```python
from build123d import *

# Parameters (mm, degrees)
SKETCH1_W           = 50
SKETCH1_H           = 40
BOSS_EXTRUDE1_DEPTH = 10
SKETCH5_W           = 6
SKETCH5_H           = 5
BOSS_EXTRUDE3_DEPTH = 10
SKETCH6_R           = 2
CUT_EXTRUDE1_DEPTH  = 20
SKETCH8_W           = 10
SKETCH8_H           = 40
CUT_EXTRUDE2_DEPTH  = 25
SKETCH9_W           = 10
SKETCH9_H           = 6
SKETCH9_R           = 1.25
BOSS_EXTRUDE4_DEPTH = 5
SKETCH10_W          = 10
SKETCH10_H          = 5
CUT_EXTRUDE3_DEPTH  = 15
SKETCH11_W          = 5
SKETCH11_H          = 5
BOSS_EXTRUDE5_DEPTH = 10
SKETCH12_R          = 1.25
CUT_EXTRUDE4_DEPTH  = 10
CUT_EXTRUDE5_DEPTH  = 10
CUT_EXTRUDE6_DEPTH  = 10
SCALE1_SCALE        = 2
SKETCH15_W          = 33.464905159
SKETCH15_H          = 55
SKETCH15_W_2        = 35
SKETCH15_H_2        = 25
CUT_EXTRUDE7_DEPTH  = 30


with BuildPart() as part:
    # Sketch1 → Boss-Extrude1 (new body)
    with BuildSketch(Plane(origin=(669.84184187, 0, 0), x_dir=(1, 0, 0), z_dir=(0, 0, 1))):
        with Locations((-671.310344828, 437.637931034)):
            Rectangle(SKETCH1_W, SKETCH1_H)
    boss_extrude1 = extrude(amount=BOSS_EXTRUDE1_DEPTH)

    # Sketch5 → Boss-Extrude3 (add)
    with BuildSketch(Plane(origin=(23.531497042, 0, 0), x_dir=(0, 0, -1), z_dir=(1, 0, 0))):
        with Locations((-5, 442.637931034)):
            Rectangle(SKETCH5_W, SKETCH5_H)
        with Locations((-5, 432.637931034)):
            Rectangle(SKETCH5_W, SKETCH5_H)
    extrude(amount=BOSS_EXTRUDE3_DEPTH)

    # Sketch6 → Cut-Extrude1 (cut)
    with BuildSketch(Plane(origin=(669.84184187, 445.137931034, 0), x_dir=(1, 0, 0), z_dir=(0, 1, 0))):
        with Locations(Location((-641.310344828, -5, 0), (0, 0, 180))):
            Circle(SKETCH6_R)
    extrude(amount=-CUT_EXTRUDE1_DEPTH, mode=Mode.SUBTRACT)

    # Sketch8 → Cut-Extrude2 (cut)
    with BuildSketch(Plane.ZY.offset(26.468502958)):
        with Locations((5, 437.637931034)):
            Rectangle(SKETCH8_W, SKETCH8_H)
    extrude(amount=-CUT_EXTRUDE2_DEPTH, mode=Mode.SUBTRACT)

    # Sketch9 → Boss-Extrude4 (add)
    with BuildSketch(Plane(origin=(0, 435.137931034, 0), x_dir=(1, 0, 0), z_dir=(0, 1, 0))):
        with Locations((28.531497042, -5)):
            Rectangle(SKETCH9_W, SKETCH9_H)
        with Locations(Location((28.531497042, -5, 0), (0, 0, 180))):
            Circle(SKETCH9_R, mode=Mode.SUBTRACT)
    extrude(amount=BOSS_EXTRUDE4_DEPTH)

    # Sketch10 → Cut-Extrude3 (cut)
    with BuildSketch(Plane.XY.offset(8)):
        with Locations((28.531497042, 432.637931034)):
            Rectangle(SKETCH10_W, SKETCH10_H)
        with Locations((28.531497042, 442.637931034)):
            Rectangle(SKETCH10_W, SKETCH10_H)
    extrude(amount=-CUT_EXTRUDE3_DEPTH, mode=Mode.SUBTRACT)

    # Mirror1: Boss-Extrude1 across plane
    add(boss_extrude1.mirror(Plane(origin=(-1.468502958, 0, 0), x_dir=(0, 0, 1), z_dir=(1, 0, 0))))

    # Sketch11 → Boss-Extrude5 (add)
    with BuildSketch(Plane(origin=(0, 457.637931034, 0), x_dir=(1, 0, 0), z_dir=(0, 1, 0))):
        with Locations((-1.468502958, -5)):
            Rectangle(SKETCH11_W, SKETCH11_H)
    extrude(amount=BOSS_EXTRUDE5_DEPTH)

    # Sketch12 → Cut-Extrude4 (cut)
    with BuildSketch(Plane(origin=(1.031497042, 0, 0), x_dir=(0, 0, -1), z_dir=(1, 0, 0))):
        with Locations((-5, 462.637931034)):
            Circle(SKETCH12_R)
    extrude(amount=-CUT_EXTRUDE4_DEPTH, mode=Mode.SUBTRACT)

    # Sketch13 → Cut-Extrude5 (cut)
    with BuildSketch(Plane(origin=(1.031497042, 0, 0), x_dir=(0, 0, -1), z_dir=(1, 0, 0))):
        with BuildLine():
            Line((-7.5, 467.637931034), (-7.5, 462.637931034))
            ThreePointArc((-7.5, 462.637931034), (-5, 465.137931034), (-2.5, 462.637931034))
            Line((-2.5, 462.637931034), (-2.5, 467.637931034))
            Line((-2.5, 467.637931034), (-7.5, 467.637931034))
        make_face()
    extrude(amount=-CUT_EXTRUDE5_DEPTH, mode=Mode.SUBTRACT)

    # Sketch14 → Cut-Extrude6 (cut)
    with BuildSketch(Plane(origin=(0, 440.137931034, 0), x_dir=(1, 0, 0), z_dir=(0, 1, 0))):
        with BuildLine():
            Line((33.531497042, -2), (28.531497042, -2))
            ThreePointArc((28.531497042, -2), (30.652817386, -2.878679656), (31.531497042, -5))
            ThreePointArc((31.531497042, -5), (30.652817386, -7.121320344), (28.531497042, -8))
            Line((28.531497042, -8), (33.531497042, -8))
            Line((33.531497042, -8), (33.531497042, -2))
        make_face()
    extrude(amount=-CUT_EXTRUDE6_DEPTH, mode=Mode.SUBTRACT)


with BuildPart() as part_1:
    # Scale1: scaled about (-1.193296494, 437.808884999, 5)
    add(part.part.scale(SCALE1_SCALE).moved(Location((1.193296494, -437.808884999, -5))))

    # Sketch15 → Cut-Extrude7 (cut)
    with BuildSketch(Plane.XY.offset(15)):
        with Locations((-35.011256843, 449.96697707)):
            Rectangle(SKETCH15_W, SKETCH15_H)
        Polygon((-51.743709422, 422.46697707), (-51.743709422, 397.46697707), (48.256290578, 397.46697707), (48.256290578, 422.46697707), (-18.278804263, 422.46697707), align=None)
        with Locations((30.756290578, 464.96697707)):
            Rectangle(SKETCH15_W_2, SKETCH15_H_2)
    extrude(amount=-CUT_EXTRUDE7_DEPTH, mode=Mode.SUBTRACT)


solid = part_1.part
```
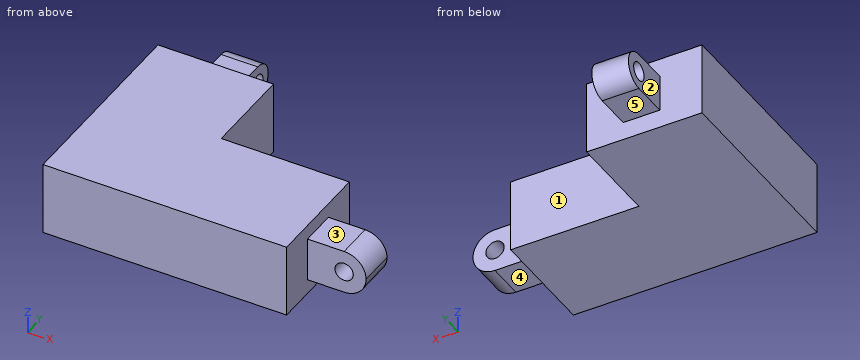
Design review of the part built by this model. Coordinates are the model's own, in mm. Face numbers are marked on the shaded views. A direction names the side the tool comes from. Coordinates: 2 decimals unless noted, no trailing zeros. Loops run counter-clockwise (first coordinate to the right, second up) from the corner with the lowest first, then second, coordinate; pieces in that order, holes last.
Q1. We need section D-D on y = 431.5. State the section outline as (x, z) points.
Reported:
outline: (-18.28, -5) - (48.26, -5) - (48.26, 15) - (-18.28, 15) - close
Q2. For pin 1 (3 mm diameter, centred on x = -2.5, y = 482.5, fed in from +Z); pin 2 (11 mm diameter, centred on x = 0, y = 483, fed in from -Z); pin 3 (11 mm diameter, centred on y = 484.5, z = 4, fed in from -X), all flat-tipped, find the tip position at first contact; note any pin that passes through.
Reported:
pin 1: stops at z = 10
pin 2: stops at z = 0
pin 3: stops at x = -6.74
Q3. We need section B-B on z = 6. State the section outline as (x, y) points (3 decimals).
Reported:
outline: (-18.279, 422.467) - (48.256, 422.467) - (48.256, 432.467) - (55.965, 432.467) - (55.965, 442.467) - (48.256, 442.467) - (48.256, 452.467) - (13.256, 452.467) - (13.256, 477.467) - (3.256, 477.467) - (3.256, 485.176) - (-6.744, 485.176) - (-6.744, 477.467) - (-18.279, 477.467) - close; (-6.744, 489.758) - (3.256, 489.758) - (3.256, 492.366) - (-6.744, 492.366) - close; (60.548, 432.467) - (64.172, 432.467) - (64.172, 442.467) - (60.548, 442.467) - close
Q4. We need section C-C on z = 12.25. State the section outline as (x, y) points.
Reported:
outline: (-18.28, 422.47) - (48.26, 422.47) - (48.26, 452.47) - (13.26, 452.47) - (13.26, 477.47) - (-18.28, 477.47) - close
Q5. Tool access review of the marked faces 1, 2, 3, 4 and 5: name each direction out of +Z, -Z, +X, -X, +Y, -Y from which nothing blocks a thin tool from reaching the whole face with its end or side.
Reported:
face 1: +Z, -Z, +X, +Y
face 2: +Z, -Z, -X, +Y
face 3: +Z, +X, +Y, -Y
face 4: -Z, +X, +Y, -Y
face 5: -Z, +X, -X, +Y
Q6. We need section A-A on x = 1. State the section outline as (y, z) points.
Reported:
outline: (422.47, -5) - (477.47, -5) - (477.47, 0) - (487.47, 0) arc R5 ccw to (487.47, 10) - (477.47, 10) - (477.47, 15) - (422.47, 15) - close; hole circle Ø5 at (487.47, 5)
Q7. To check wall thickness, follow line 1 (Y direction, x = -2.75, z = 5); line 2 (X direction, y = 477, z = -0.75); line 3 (Y direction, x = 51.5, z = 0.75). State the ranges of each line that lie inside material, in increasing order.
Reported:
line 1: y = 422.47 to 484.97, 489.97 to 492.47
line 2: x = -18.28 to 13.26
line 3: y = 432.47 to 442.47
